```python
from build123d import *

# Parameters (mm, degrees)
SKETCH_1_R          = 1.65
EXTRUDE_1_DEPTH     = 3
SKETCH_2_R          = 5.5
EXTRUDE_2_DEPTH     = 1.5
CUT_EXTRUDE_1_DEPTH = 0.8
FILLET_1_R          = 17


with BuildPart() as part:
    # 草图1 → 凸台-拉伸1 (new body)
    with BuildSketch(Plane.XY):
        with BuildLine():
            Line((-5.08774827, -1.216070925), (0.41225173, -15.716070925))
            ThreePointArc((0.41225173, -15.716070925), (4.301339026, -25.105158222), (-5.08774827, -21.216070925))
            Line((-5.08774827, -21.216070925), (-12.673955167, -1.216070925))
            Line((-12.673955167, -1.216070925), (-5.08774827, 18.783929075))
            ThreePointArc((-5.08774827, 18.783929075), (4.301339026, 22.673016371), (0.41225173, 13.283929075))
            Line((0.41225173, 13.283929075), (-5.08774827, -1.216070925))
        make_face()
        with Locations((0.41225173, -21.216070925)):
            Circle(SKETCH_1_R, mode=Mode.SUBTRACT)
        with Locations(Location((0.41225173, 18.783929075, 0), (0, 0, 180))):
            Circle(SKETCH_1_R, mode=Mode.SUBTRACT)
    extrude(amount=EXTRUDE_1_DEPTH)

    # 草图2 → 凸台-拉伸2 (add)
    # profile 1 of 2: a face of its own
    with BuildSketch(Plane.XY.offset(3)):
        with Locations(Location((0.41225173, 18.783929075, 0), (0, 0, 180))):
            Circle(SKETCH_2_R)
        Polygon((-2.48774827, 20.458244856), (-2.48774827, 17.109613294), (0.41225173, 15.435297514), (3.31225173, 17.109613294), (3.31225173, 20.458244856), (0.41225173, 22.132560636), align=None, mode=Mode.SUBTRACT)
    # profile 2 of 2: a face of its own
    with BuildSketch(Plane.XY.offset(3)):
        with Locations(Location((0.41225173, -21.216070925, 0), (0, 0, 180))):
            Circle(SKETCH_2_R)
        Polygon((-2.48774827, -19.541755144), (-2.48774827, -22.890386706), (0.41225173, -24.564702486), (3.31225173, -22.890386706), (3.31225173, -19.541755144), (0.41225173, -17.867439364), align=None, mode=Mode.SUBTRACT)
    extrude(amount=EXTRUDE_2_DEPTH)

    # 草图3 → 切除-拉伸1 (cut)
    with BuildSketch(Plane.XY.offset(3)):
        Polygon((0.41225173, 22.132560636), (-2.48774827, 20.458244856), (-2.48774827, 17.109613294), (0.41225173, 15.435297514), (3.31225173, 17.109613294), (3.31225173, 20.458244856), align=None)
        Polygon((0.41225173, -17.867439364), (-2.48774827, -19.541755144), (-2.48774827, -22.890386706), (0.41225173, -24.564702486), (3.31225173, -22.890386706), (3.31225173, -19.541755144), align=None)
    extrude(amount=-CUT_EXTRUDE_1_DEPTH, mode=Mode.SUBTRACT)

    # 圆角1
    # the kernel refuses this fillet: 17 mm, written as the material it adds along each edge
    with BuildSketch(Plane(origin=(-5.08774827, 18.783929075, 0), x_dir=(0.09189054947258435, 0.9957691132574993, 0), z_dir=(0, 0, 1))) as fillet_1_piece_1:
        with BuildLine():
            CenterArc((2.572935385, 16.928074925), FILLET_1_R, 254.500123691, 10.227497936)
            Line((-1.970081643, 0.546347413), (0, 0))
            ThreePointArc((0, 0), (0.505398022, 0.023269877), (1.010796044, 0))
        make_face()
    extrude(amount=3)
    with BuildSketch(Plane(origin=(0.41225173, 13.283929075, 0), x_dir=(-0.3546542341205386, -0.9349975263177835, 0), z_dir=(0, 0, 1))) as fillet_1_piece_2:
        with BuildLine():
            CenterArc((6.987015843, 17), FILLET_1_R, 237.378356152, 32.621643848)
            ThreePointArc((-2.177496959, 2.681770183), (-0.872736529, 1.516278705), (0, 0))
            Line((0, 0), (6.987015843, 0))
        make_face()
    extrude(amount=3)
    with BuildSketch(Plane(origin=(-5.08774827, -1.216070925, 0), x_dir=(0.35465423412053854, 0.9349975263177835, 0), z_dir=(0, 0, 1))) as fillet_1_piece_3:
        with BuildLine():
            CenterArc((FILLET_1_R * 0.379310344828, -FILLET_1_R), FILLET_1_R, 90, 41.544509364)
            Line((-FILLET_1_R * 0.283891318374, -FILLET_1_R * 0.251559251559), (0, 0))
            Line((0, 0), (FILLET_1_R * 0.379310344828, 0))
        make_face()
    extrude(amount=3)
    with BuildSketch(Plane(origin=(0.41225173, -15.716070925, 0), x_dir=(-0.35465423412053854, 0.9349975263177834, 0), z_dir=(0, 0, 1))) as fillet_1_piece_4:
        with BuildLine():
            CenterArc((6.987015843, -17), FILLET_1_R, 90, 32.621643848)
            ThreePointArc((-2.177496959, -2.681770183), (-0.872736529, -1.516278705), (0, 0))
            Line((0, 0), (6.987015843, 0))
        make_face()
    extrude(amount=3)
    with BuildSketch(Plane(origin=(-5.08774827, -21.216070925, 0), x_dir=(0.09189054947258435, -0.9957691132574993, 0), z_dir=(0, 0, 1))) as fillet_1_piece_5:
        with BuildLine():
            CenterArc((2.572935385, -16.928074925), FILLET_1_R, 95.272378373, 10.227497936)
            Line((-1.970081643, -0.546347413), (0, 0))
            ThreePointArc((0, 0), (0.505398022, -0.023269877), (1.010796044, 0))
        make_face()
    extrude(amount=3)
    # the kernel refuses this fillet: 17 mm, written as the material it takes off along each edge
    with BuildSketch(Plane(origin=(-12.673955167, -1.216070925, -16.120689655), x_dir=(0.35465423412053854, 0.9349975263177835, 0), z_dir=(0, 0, 1))) as fillet_1_2_piece_1:
        with BuildLine():
            CenterArc((FILLET_1_R * 0.379310344828, -FILLET_1_R), FILLET_1_R, 90, 41.544509364)
            Line((-FILLET_1_R * 0.283891318374, -FILLET_1_R * 0.251559251559), (0, 0))
            Line((0, 0), (FILLET_1_R * 0.379310344828, 0))
        make_face()
    extrude(amount=35.24137931, mode=Mode.SUBTRACT)


solid = part.part
```
Verification items for the finished model (mm, model axes). A direction names the side the tool comes from. Give positions to 0.01 mm unless a question says otherwise; leave off trailing zeros. Loops run counter-clockwise (first coordinate to the right, second up) from the corner with the lowest first, then second, coordinate; pieces in that order, holes last. Notation, with made-up numbers: M -29,13.25 L -14,13.25 A14 cw -14,31.25 Z; hole C 42.25,68 d11. An arc over 180 degrees is marked long. Return JSON: item names as keys, results as strings.
1) Section check D-D, the plane z = 1.75. Enter the section's corners in (x, y).
Findings:
{"outline": "M -10.39,-7.25 L -5.81,-19.3 A17 cw -4.99,-22.22 A5.5 ccw long 3.69,-16.8 A17 cw -2.07,-9.18 L -2.8,-7.25 A17 cw -2.8,4.81 L -2.07,6.75 A17 cw 3.69,14.37 A5.5 ccw long -4.99,19.79 A17 cw -5.81,16.87 L -10.39,4.81 A17 ccw Z; hole C 0.41,-21.22 d3.3; hole C 0.41,18.78 d3.3"}
2) Tool access check on faces 1 (the cylindrical face through (0.31, 11.03, 1.48)), 2 (the flat face through (-6, -2, 0)), 3 (the flat face through (-2.488, 19, 3)). Record the directions out of +Z, -Z, +X, -X, +Y, -Y that give a thin tool (end or side, any length) a straight path to the whole face; none if there is none.
Findings:
{"face 1": "+Z, -Z, +X", "face 2": "-Z, +X, -X, +Y, -Y", "face 3": "+Z"}
3) Section check C-C, the plane y = 21. Enter the section's corners in (x, z), and give its area (3 significant figures).
Findings:
{"outline": "M -4.62,0 L 5.45,0 L 5.45,4.5 L 2.37,4.5 L 2.37,2.2 L -1.55,2.2 L -1.55,4.5 L -4.62,4.5 Z", "area": "36.3 mm2"}
4) Section check A-A, the plane z = 3.75. Enter the section's corners in (x, y), and give its area (3 significant figures).
Findings:
{"outline": "C 0.41,-21.22 d11; C 0.41,18.78 d11; hole M -2.49,-22.89 L 0.41,-24.56 L 3.31,-22.89 L 3.31,-19.54 L 0.41,-17.87 L -2.49,-19.54 Z; hole M -2.49,17.11 L 0.41,15.44 L 3.31,17.11 L 3.31,20.46 L 0.41,22.13 L -2.49,20.46 Z", "area": "132 mm2"}
5) Material ranges on L1, parallel to Y at x = 1.5, z = 4; L2, parallel to Y at x = 0.5, z = 4.35; L3, parallel to Z at x = -4.25, y = -10, recorded low to high. Write a range as [from, to].
Findings:
{"L1": "y = [-26.61, -23.94], [-18.5, -15.82], [13.39, 16.06], [21.5, 24.18]", "L2": "y = [-26.72, -24.51], [-17.92, -15.72], [13.28, 15.49], [22.08, 24.28]", "L3": "z = [0, 3]"}
6) Section check B-B, the plane x = 2.75. Enter the section's corners in (y, z) (3 decimals), and give its area (3 significant figures).
Findings:
{"outline": "M -26.195,0 L -16.048,0 L -16.048,3 L -16.238,3 L -16.238,4.5 L -19.217,4.5 L -19.217,2.2 L -23.215,2.2 L -23.215,4.5 L -26.195,4.5 Z; M 13.616,0 L 23.762,0 L 23.762,4.5 L 20.783,4.5 L 20.783,2.2 L 16.785,2.2 L 16.785,4.5 L 13.805,4.5 L 13.805,3 L 13.616,3 Z", "area": "72.4 mm2"}
7) Mould release check, pull along X, two halves, no side actions. Record for faces 4 (the flat face through (-5, -2, 3)), 5 (the cylindrical face through (-0.47, 17.39, 1.08)), 6 (the cylindrical face through (-5.33, -20.77, 1.48)): released by +X, released by -X, zero draft, split by the parting line, or undercut.
Findings:
{"face 4": "zero draft", "face 5": "undercut", "face 6": "released by -X"}
8) Gauge pin test, flat ends, axial feed: P1, Ø2.5, axis at y = -21.5, z = 3.5, coming from the -X side; P2, Ø8, axis at x = -6.5, y = -14, coming from the +Z side; P3, Ø1, axis at x = -2, z = 0.5, coming from the -Y side; P4, Ø2.5, axis at x = 0.41, y = 18.78, coming from the -Z side. Record the tip position at first contact, or that the pin passes through.
Findings:
{"P1": "stops at x = -5.45", "P2": "stops at z = 3", "P3": "stops at y = -26.37", "P4": "passes through"}
